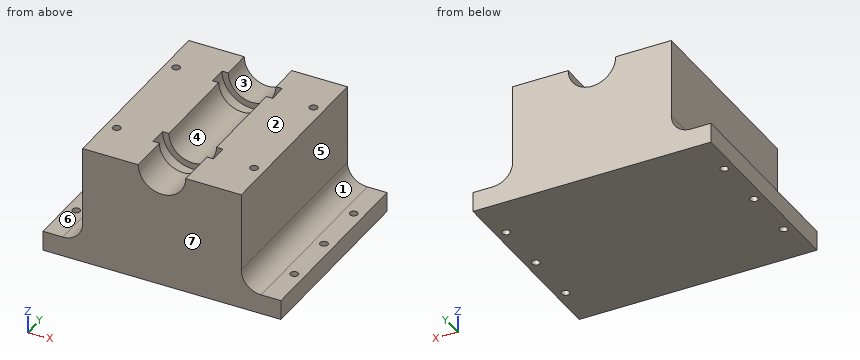
from build123d import *

# Parameters (mm, degrees)
F0_W      = 60
F0_H      = 50
F1_DEPTH  = 30
F3_R      = 6
F4_DEPTH  = 90
F6_R      = 7.6
F7_DEPTH  = 4.5
F8_START  = -28
F8_DEPTH  = 4.5
F10_R     = 1
F11_DEPTH = 25
F12_R     = 1
F13_DEPTH = 5


with BuildPart() as f1:
    # F0 (on Top) → F1 (new body)
    with BuildSketch(Plane.XY):
        with Locations((-8.3905272186, 29.4691909945)):
            Rectangle(F0_W, F0_H)
    extrude(amount=F1_DEPTH)

    # F3 (on face) → F4 (cut)
    with BuildSketch(Plane.XZ.offset(-4.4691909945)):
        with Locations((-8.3905272186, 30)):
            Circle(F3_R)
        with BuildLine():
            Line((-28.3905272186, 10), (-28.3905272186, 30))
            Line((-28.3905272186, 30), (-38.3905272186, 30))
            Line((-38.3905272186, 30), (-38.3905272186, 5))
            Line((-38.3905272186, 5), (-33.3905272186, 5))
            ThreePointArc((-33.3905272186, 5), (-29.8549933126, 6.4644660941), (-28.3905272186, 10))
        make_face()
        with BuildLine():
            Line((21.6094727814, 5), (21.6094727814, 30))
            Line((21.6094727814, 30), (11.6094727814, 30))
            Line((11.6094727814, 30), (11.6094727814, 10))
            ThreePointArc((11.6094727814, 10), (13.0739388755, 6.4644660941), (16.6094727814, 5))
            Line((16.6094727814, 5), (21.6094727814, 5))
        make_face()
    extrude(amount=-F4_DEPTH, mode=Mode.SUBTRACT)

    # F6 (on offset) → F7 (cut)
    with BuildSketch(Plane.XZ.offset(-14.4691909945)):
        with Locations((-8.3905272186, 30)):
            Circle(F6_R)
    extrude(amount=-F7_DEPTH, mode=Mode.SUBTRACT)

    # F6 (on offset) → F8 (cut)
    with BuildSketch(Plane.XZ.offset(-14.4691909945).offset(F8_START)):
        with Locations((-8.3905272186, 30)):
            Circle(F6_R)
    extrude(amount=-F8_DEPTH, mode=Mode.SUBTRACT)

    # F10 (on face) → F11 (cut)
    with BuildSketch(Plane.XY.offset(5)):
        with Locations((19.1094727814, 15.4691909945)):
            Circle(F10_R)
        with Locations((19.1094727814, 43.4691909945)):
            Circle(F10_R)
        with Locations((19.1094727814, 29.4691909945)):
            Circle(F10_R)
        with Locations((-35.8905272186, 15.4691909945)):
            Circle(F10_R)
        with Locations((-35.8905272186, 29.4691909945)):
            Circle(F10_R)
        with Locations((-35.8905272186, 43.4691909945)):
            Circle(F10_R)
    extrude(amount=-F11_DEPTH, mode=Mode.SUBTRACT)

    # F12 (on face) → F13 (cut)
    with BuildSketch(Plane.XY.offset(30)):
        with Locations((8.9574727814, 43.4691909945)):
            Circle(F12_R)
        with Locations((8.9574727814, 15.4691909945)):
            Circle(F12_R)
        with Locations((-25.6856481384, 15.4691909945)):
            Circle(F12_R)
        with Locations((-25.6856481384, 43.4691909945)):
            Circle(F12_R)
    extrude(amount=-F13_DEPTH, mode=Mode.SUBTRACT)


solid = f1.part
Geometry: final body of the model. Coordinates: model frame, mm. Face numbers are marked on the shaded views. A direction names the side the tool comes from. Round coordinates to 2 decimals unless told otherwise and drop trailing zeros. Loops run counter-clockwise (first coordinate to the right, second up) from the corner with the lowest first, then second, coordinate; pieces in that order, holes last. Notation, with made-up numbers: (-36.5, 61.25) - (-4.5, 61.25) arc R18 cw to (-4.5, 81.25) - close; hole circle Ø9 at (-23, -7). An arc over 180 degrees is marked (long way). Write each question's results on one line, items separated by ' | '. Start each with the question number.
1) Cut plane D-D on z = 12. Return loops of the section in (x, y).
2) Mould query, pull axis X, two halves, no side actions, for the marked faces 1, 2, 3 and 4. Classes: released by +X, released by -X, zero draft, split by the parting line, or undercut.
3) Line query: probe 1 along X at (y, z) = (48, 14); probe 2 along Z at (x, y) = (-11, 8); probe 3 along Z at (x, y) = (17.5, 34). Output: solid intervals per line, ascending. Write a range as [from, to].
4) Cut plane C-C on x = -12. Return loops of the section in (y, z), then the cut area to 3 significant figures.
5) First-contact query: P1, Ø0.6, axis at x = 9.5, y = 43.5, coming from the +Z side; P2, Ø3, axis at y = 40, z = 12, coming from the -X side; P3, Ø2.5, axis at x = 19, y = 19, coming from the +Z side. Flat tips, straight axial feed; report the tip coordinate or a pass-through.
6) Access query for the marked faces 5, 6 and 7. Directions: +Z, -Z, +X, -X, +Y, -Y. A direction counts if a zero-diameter tool reaches every point of the face in a straight line with its end or side. Return the directions, or none.
7) Cut plane B-B on y = 13.5. Return loops of the section in (x, z).
8) Cut plane A-A on z = 26.25. Return loops of the section in (x, y).
Verdict:
1) outline: (-28.39, 4.47) - (11.61, 4.47) - (11.61, 54.47) - (-28.39, 54.47) - close
2) face 1: released by +X | face 2: zero draft | face 3: undercut | face 4: undercut
3) probe 1: x = [-28.39, 11.61] | probe 2: z = [0, 24.6] | probe 3: z = [0, 5]
4) outline: (4.47, 0) - (54.47, 0) - (54.47, 25.21) - (46.97, 25.21) - (46.97, 23.31) - (42.47, 23.31) - (42.47, 25.21) - (18.97, 25.21) - (18.97, 23.31) - (14.47, 23.31) - (14.47, 25.21) - (4.47, 25.21) - close | area: 1,240 mm2
5) P1: stops at z = 25 | P2: stops at x = -28.39 | P3: stops at z = 5
6) face 5: +Z, +X, +Y, -Y | face 6: +Z, -X, +Y, -Y | face 7: +Z, -Z, +X, -X, -Y
7) outline: (-38.39, 0) - (21.61, 0) - (21.61, 5) - (16.61, 5) arc R5 cw to (11.61, 10) - (11.61, 30) - (-2.39, 30) arc R6 cw to (-14.39, 30) - (-28.39, 30) - (-28.39, 10) arc R5 cw to (-33.39, 5) - (-38.39, 5) - close
8) outline: (-28.39, 4.47) - (-13.07, 4.47) - (-13.07, 14.47) - (-15, 14.47) - (-15, 18.97) - (-13.07, 18.97) - (-13.07, 42.47) - (-15, 42.47) - (-15, 46.97) - (-13.07, 46.97) - (-13.07, 54.47) - (-28.39, 54.47) - close; (-3.71, 4.47) - (11.61, 4.47) - (11.61, 54.47) - (-3.71, 54.47) - (-3.71, 46.97) - (-1.78, 46.97) - (-1.78, 42.47) - (-3.71, 42.47) - (-3.71, 18.97) - (-1.78, 18.97) - (-1.78, 14.47) - (-3.71, 14.47) - close; hole circle Ø2 at (-25.69, 15.47); hole circle Ø2 at (-25.69, 43.47); hole circle Ø2 at (8.96, 15.47); hole circle Ø2 at (8.96, 43.47)
